For this review, use the dimensioned drawing (mm, ordinates from the lowest corner) and the shaded views. A direction names the side the tool comes from. Round coordinates to 2 decimals unless told otherwise and drop trailing zeros. Order: outer loops, then holes, each group sorted by start corner. A loop starts at its lowest first (then second) coordinate and runs counter-clockwise, first axis right, second up. Notation, with made-up numbers: (40.25, -22.75) - (69.25, -22.75) arc R34 cw to (69.25, 8.25) - close; hole circle Ø8 at (-32.75, 12). An arc over 180 degrees is marked (long way). Write item = value, one per line.
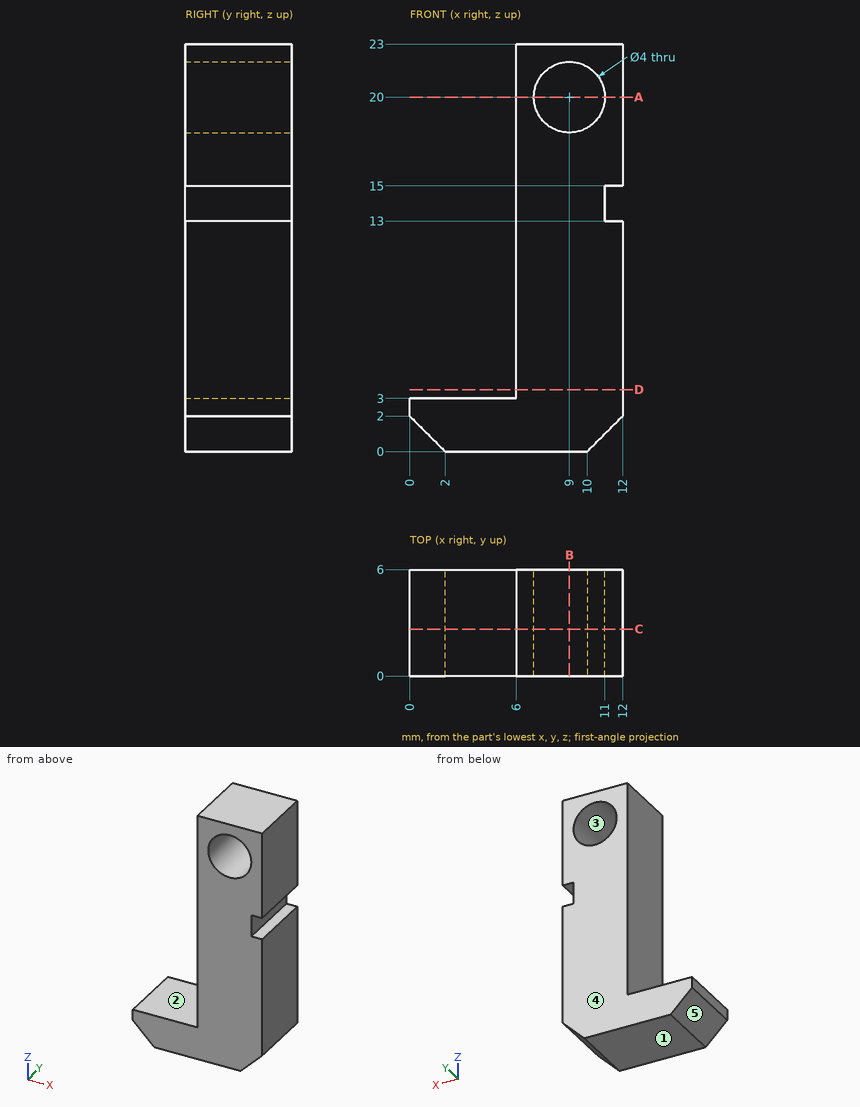
1) For the marked faces 1 and 2, list the 3-axis set-ups (+Z, -Z, +X, -X, +Y, -Y) from which the entire face can be reached by the end or side of a thin tool; tool diameter is ignored.
Findings:
face_1 = -Z, +X, -X, +Y, -Y
face_2 = +Z, -X, +Y, -Y
2) The part is to be moulded in two halves that separate along Z. For the marked faces 3, 4 and 5, say which applies: released by +Z, released by -Z, zero draft, split by the parting line, or undercut.
Findings:
face_3 = undercut
face_4 = zero draft
face_5 = released by -Z
3) We need section C-C on y = 2.65. Write out the cut boundary in (x, z).
Findings:
outline = (0, 2) - (2, 0) - (10, 0) - (12, 2) - (12, 13) - (11, 13) - (11, 15) - (12, 15) - (12, 23) - (6, 23) - (6, 3) - (0, 3) - close; hole circle Ø4 at (9, 20)
4) Clearance check with flat-ended pins moving along their axes: pin 1 Ø1.1 at (x, y) = (11.5, 1.5) entering from -Z; pin 2 Ø3.5 at (x, z) = (9, 20) entering from -Y; pin 3 Ø1.8 at (x, y) = (2, 4) entering from +Z. State where each tip first meets the part, or that it passes through.
Findings:
pin_1 = 0.95
pin_2 = through
pin_3 = 3
5) To check wall thickness, follow L1, parallel to Z at x = 9, y = 3.3; L2, parallel to X at y = 4.4, z = 20; L3, parallel to X at y = 2.5, z = 17.5. State the ranges of each line that lie inside material, in increasing order. Write a range as from..to.
Findings:
L1 = 0..18, 22..23
L2 = 6..7, 11..12
L3 = 6..12
6) We need section B-B on x = 9. Write out the cut boundary in (y, z), and give its area (3 significant figures).
Findings:
outline = (0, 0) - (6, 0) - (6, 18) - (0, 18) - close; (0, 22) - (6, 22) - (6, 23) - (0, 23) - close
area = 114 mm^2
7) We need section D-D on z = 3.5. Write out the cut boundary in (x, y), and give its area (3 significant figures).
Findings:
outline = (6, 0) - (12, 0) - (12, 6) - (6, 6) - close
area = 36.0 mm^2
8) We need section A-A on z = 20. Write out the cut boundary in (x, y).
Findings:
outline = (6, 0) - (7, 0) - (7, 6) - (6, 6) - close; (11, 0) - (12, 0) - (12, 6) - (11, 6) - close
